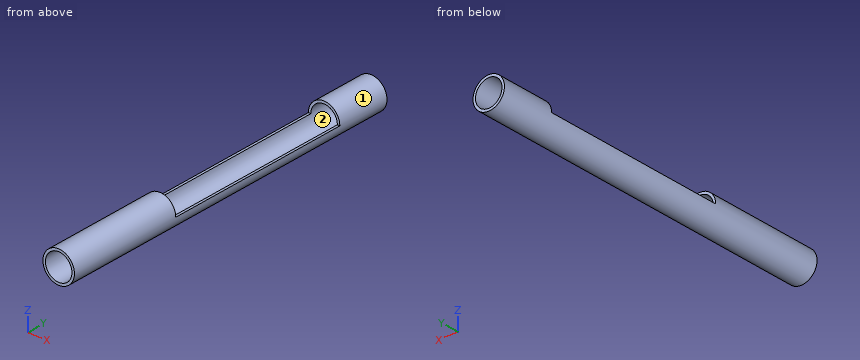
```python
from build123d import *

# Parameters (mm, degrees)
F0_R     = 13.335
F1_DEPTH = 304.8
F2_R     = 11.2268
F3_DEPTH = 304.801
F5_W     = 26.67
F5_H     = 160
F6_DEPTH = 13.335


with BuildPart() as f1:
    # F0 (on Front) → F1 (new body)
    with BuildSketch(Plane.XZ):
        Circle(F0_R)
    extrude(amount=F1_DEPTH)

    # F2 (on face) → F3 (cut, through all)
    with BuildSketch(Plane.XZ.offset(304.8)):
        Circle(F2_R)
    extrude(amount=-F3_DEPTH, mode=Mode.SUBTRACT)

    # F5 (on offset) → F6 (cut)
    with BuildSketch(Plane.XY.offset(13.335)):
        with Locations((0, -126)):
            Rectangle(F5_W, F5_H)
    extrude(amount=-F6_DEPTH, mode=Mode.SUBTRACT)


solid = f1.part
```
The model under review builds one solid part; all positions refer to its coordinate system, in mm. Face numbers are marked on the shaded views. Give positions to 0.01 mm unless a question says otherwise; leave off trailing zeros. Write each loop counter-clockwise with the first axis right and the second up, starting at its lowest first coordinate (ties: lowest second). Pieces come first, ordered by that corner, then holes. Notation, with made-up numbers: (22.5, 45.25) -> (37.5, 45.25) arc R11 cw to (37.5, 63.25) -> close; hole circle Ø8 at (-21.5, 60). An arc over 180 degrees is marked (long way). Answer in a Markdown table with one row per item.
1) Clearance check with flat-ended pins moving along their axes: P1, Ø1.5, axis at x = 0.5, y = -90.5, coming from the +Z side; P2, Ø3, axis at x = -2.5, z = -9, coming from the +Y side; P3, Ø10, axis at x = -6.5, y = -239.5, coming from the +Z side; P4, Ø1.1, axis at x = -12.5, y = -151.5, coming from the +Z side. State where each tip first meets the part, or that it passes through.
Worked answers:
| item | result |
|---|---|
| P1 | z = -11.16 |
| P2 | through |
| P3 | z = 13.25 |
| P4 | z = 0 |
2) Mouldability with a two-part tool opening along Z and no side actions: class the marked faces 1 and 2 as +Z half, -Z half, draft (parallel to the pull), parting line (faces both ways), or undercut.
Worked answers:
| item | result |
|---|---|
| face 1 | parting line |
| face 2 | undercut |
3) Add section B-B on z = -5. State the section outline as (x, y) points, plus the area to 3 significant figures.
Worked answers:
| item | result |
|---|---|
| outline | (-12.36, -304.8) -> (-10.05, -304.8) -> (-10.05, 0) -> (-12.36, 0) -> close; (10.05, -304.8) -> (12.36, -304.8) -> (12.36, 0) -> (10.05, 0) -> close |
| area | 1,410 mm² |
4) Add section C-C on y = -254. State the section outline as (x, z) points (3 decimals), plus the area to 3 significant figures.
Worked answers:
| item | result |
|---|---|
| outline | circle Ø26.67 at (0, 0); hole circle Ø22.454 at (0, 0) |
| area | 163 mm² |
5) For L1, parallel to Y at x = -0.5, z = 12.25; L2, parallel to X at y = -238, z = 0 (3 decimals); L3, parallel to Z at x = 0, y = -95 (3 decimals), list the stretches that pass through material, from the lowest coordinate up. Write a range as [from, to].
Worked answers:
| item | result |
|---|---|
| L1 | [-304.8, -206], [-46, 0] |
| L2 | [-13.335, -11.227], [11.227, 13.335] |
| L3 | [-13.335, -11.227] |
6) Add section A-A on x = 0. State the section outline as (y, z) points (3 decimals), plus the area to 3 significant figures.
Worked answers:
| item | result |
|---|---|
| outline | (-304.8, -13.335) -> (0, -13.335) -> (0, -11.227) -> (-304.8, -11.227) -> close; (-304.8, 11.227) -> (-206, 11.227) -> (-206, 13.335) -> (-304.8, 13.335) -> close; (-46, 11.227) -> (0, 11.227) -> (0, 13.335) -> (-46, 13.335) -> close |
| area | 948 mm² |
7) Add section D-D on y = -108.5. State the section outline as (x, z) points (3 decimals).
Worked answers:
| item | result |
|---|---|
| outline | (-13.335, 0) arc R13.335 ccw to (13.335, 0) -> (11.227, 0) arc R11.227 cw to (-11.227, 0) -> close |
